Source: CAD feature listing. Evaluate the final solid. Frame: model axes, mm. Round coordinates to 2 decimals unless told otherwise and drop trailing zeros. Order: outer loops, then holes, each group sorted by start corner. A loop starts at its lowest first (then second) coordinate and runs counter-clockwise, first axis right, second up. Notation, with made-up numbers: M -12,5 L 39,5 A16 ccw 39,25 Z; hole C -12,47 d7. An arc over 180 degrees is marked long. Answer as CSV lines item,"result". Start each with the question number.
Item 1: Section query C-C on x = -110.5. Return the cut outline in (y, z), plus the area to 3 significant figures.
Item 2: Section query A-A on x = -41. Return the cut outline in (y, z), plus the area to 3 significant figures.
Item 3: Section query B-B on z = -5. Return the cut outline in (x, y), plus the area to 3 significant figures.
Item 4: First-contact query: P1, Ø3, axis at x = -23.5, z = 85, coming from the +Y side. Flat tip, straight axial feed; report the tip coordinate or a pass-through.
Item 5: Line query: line 1 (X direction, y = -2.25, z = 72); line 2 (X direction, y = -0.65, z = 65); line 3 (Z direction, x = -73, y = -1.25). Output: solid intervals per line, ascending. Write a range as [from, to].
from build123d import *

# Parameters (mm, degrees)
F1_DEPTH = 3
F2_DEPTH = 25
F3_R     = 20
F4_R     = 100
F5_R     = 15


with BuildPart() as f1:
    # F0 (on Front) → F1 (new body)
    with BuildSketch(Plane.XZ):
        with BuildLine():
            ThreePointArc((-119.2295857728, 16.5976797057), (-89.2269882152, -21.8866064143), (-44.5863344816, -2.1785326218))
            ThreePointArc((-44.5863344816, -2.1785326218), (-31.5003837254, 22.7075657451), (-18.8527258188, 47.819251244))
            ThreePointArc((-18.8527258187, 47.819251244), (-11.5073907558, 58.7139707042), (-8.9261215756, 71.5975225717))
            Line((-8.9261215756, 71.5975225717), (-11.67442069, 71.5975225717))
            Line((-11.67442069, 71.5975225717), (-11.67442069, 74.0203762137))
            ThreePointArc((-11.67442069, 74.0203762137), (-14.431706638, 81.8781100982), (-19.1607128584, 88.7325325952))
            ThreePointArc((-19.1607128584, 88.7325325952), (-48.5320541227, 98.3962580043), (-71.9061774941, 78.1548738354))
            Line((-71.9061774941, 78.1548738354), (-107.2845857728, 78.1548738354))
            Line((-107.2845857728, 78.1548738354), (-119.2295857728, 78.1548738354))
            Line((-119.2295857728, 78.1548738354), (-119.2295857728, 66.2098738354))
            Line((-119.2295857728, 66.2098738354), (-119.2295857728, 16.5976797057))
        make_face()
        with BuildLine():
            ThreePointArc((-26.6928125913, 79.0930187933), (-24.6315082315, 75.5227380173), (-23.3711215756, 71.597523888))
            Line((-23.3711215756, 71.597523888), (-20.8711215756, 71.5975236602))
            ThreePointArc((-20.8711215756, 71.5975236602), (-22.8939959961, 62.4935676044), (-28.5819229469, 55.1029300277))
            ThreePointArc((-28.5819229469, 55.1029300277), (-41.6104278008, 29.1671780434), (-55.1096433175, 3.4732809051))
            ThreePointArc((-55.1096433175, 3.4732809051), (-86.3130475025, -10.3024804429), (-107.2845857728, 16.5976797057))
            Line((-107.2845857728, 16.5976797057), (-107.2845857728, 66.2098738354))
            Line((-107.2845857728, 66.2098738354), (-104.7845857728, 66.2098738354))
            Line((-104.7845857728, 66.2098738354), (-68.5864427672, 66.2098738354))
            Line((-68.5864427672, 66.2098738354), (-63.1803487139, 66.2098738354))
            ThreePointArc((-63.1803487139, 66.2098738354), (-63.6941147242, 68.8812286524), (-63.8664115811, 71.5960777945))
            Line((-63.8664115811, 71.5960777945), (-61.3664115868, 71.5962461646))
            ThreePointArc((-61.3664115868, 71.5962461646), (-46.4685424734, 86.625019162), (-26.6928125913, 79.0930187933))
        make_face(mode=Mode.SUBTRACT)
        with BuildLine():
            ThreePointArc((-32.7025071715, 52.3956462756), (-51.243606048, 52.0172813271), (-63.1803487139, 66.2098738354))
            Line((-63.1803487139, 66.2098738354), (-68.5864427672, 66.2098738354))
            Line((-68.5864427672, 66.2098738354), (-104.7845857728, 66.2098738354))
            Line((-104.7845857728, 66.2098738354), (-104.7845857728, 16.5976797057))
            ThreePointArc((-104.7845857728, 16.5976797057), (-85.7031813006, -7.8780087034), (-57.3120938901, 4.6561636023))
            ThreePointArc((-57.3120938901, 4.6561636023), (-44.8056231456, 28.4219407394), (-32.7025071715, 52.3956462756))
        make_face()
        with BuildLine():
            ThreePointArc((-61.3664115868, 71.5962461646), (-42.368127741, 52.5998806027), (-23.3711215756, 71.597523888))
            Line((-23.3711215756, 71.597523888), (-28.5062876117, 71.7030383349))
            ThreePointArc((-28.5062876117, 71.7030383349), (-35.0280474509, 67.9936357913), (-42.4162418185, 66.6868830916))
            ThreePointArc((-42.4162418185, 66.6868830916), (-49.8149115034, 67.9342855665), (-56.3664115867, 71.5913571683))
            Line((-56.3664115866, 71.5913571683), (-61.3664115868, 71.5962461646))
        make_face()
        with BuildLine():
            ThreePointArc((-55.1096433175, 3.4732809051), (-41.6104278008, 29.1671780434), (-28.5819229469, 55.1029300277))
            ThreePointArc((-28.5819229469, 55.1029300277), (-30.5643455059, 53.6307678626), (-32.7025071715, 52.3956462756))
            ThreePointArc((-32.7025071715, 52.3956462756), (-44.8056231456, 28.4219407394), (-57.3120938901, 4.6561636023))
            ThreePointArc((-57.3120938901, 4.6561636023), (-85.7031813006, -7.8780087034), (-104.7845857728, 16.5976797057))
            Line((-104.7845857728, 16.5976797057), (-104.7845857728, 66.2098738354))
            Line((-104.7845857728, 66.2098738354), (-107.2845857728, 66.2098738354))
            Line((-107.2845857728, 66.2098738354), (-107.2845857728, 16.5976797057))
            ThreePointArc((-107.2845857728, 16.5976797057), (-86.3130475025, -10.3024804429), (-55.1096433175, 3.4732809051))
        make_face()
        with BuildLine():
            ThreePointArc((-42.4162418185, 66.6868830916), (-35.0280474509, 67.9936357913), (-28.5062876117, 71.7030383349))
            ThreePointArc((-28.5062876117, 71.7030383349), (-42.4756351565, 81.447422187), (-56.3664115866, 71.5913571682))
            ThreePointArc((-56.3664115867, 71.5913571683), (-49.8149115034, 67.9342855665), (-42.4162418185, 66.6868830916))
        make_face()
        with BuildLine():
            Line((-28.5062876117, 71.7030383349), (-23.3711215756, 71.597523888))
            ThreePointArc((-23.3711215756, 71.597523888), (-24.6315082315, 75.5227380173), (-26.6928125913, 79.0930187933))
            ThreePointArc((-26.6928125913, 79.0930187933), (-46.4685424734, 86.625019162), (-61.3664115868, 71.5962461646))
            Line((-61.3664115868, 71.5962461646), (-56.3664115866, 71.5913571683))
            ThreePointArc((-56.3664115866, 71.5913571682), (-42.4756351565, 81.447422187), (-28.5062876117, 71.7030383349))
        make_face()
        with BuildLine():
            Line((-20.8711215756, 71.5975236602), (-23.3711215756, 71.597523888))
            ThreePointArc((-23.3711215756, 71.597523888), (-42.368127741, 52.5998806027), (-61.3664115868, 71.5962461646))
            Line((-61.3664115868, 71.5962461646), (-63.8664115811, 71.5960777945))
            ThreePointArc((-63.8664115811, 71.5960777945), (-63.6941147242, 68.8812286524), (-63.1803487139, 66.2098738354))
            ThreePointArc((-63.1803487139, 66.2098738354), (-51.243606048, 52.0172813271), (-32.7025071715, 52.3956462756))
            ThreePointArc((-32.7025071715, 52.3956462756), (-30.5643455059, 53.6307678626), (-28.5819229469, 55.1029300277))
            ThreePointArc((-28.5819229469, 55.1029300277), (-22.8939959961, 62.4935676044), (-20.8711215756, 71.5975236602))
        make_face()
        with BuildLine():
            Line((-11.67442069, 71.5975225717), (-8.9261215756, 71.5975225717))
            ThreePointArc((-8.9261215756, 71.5975225717), (-13.1797411051, 80.6808937541), (-19.1607128584, 88.7325325952))
            ThreePointArc((-19.1607128584, 88.7325325952), (-14.431706638, 81.8781100982), (-11.67442069, 74.0203762137))
            Line((-11.67442069, 74.0203762137), (-11.67442069, 71.5975225717))
        make_face()
    extrude(amount=F1_DEPTH)

    # F0 (on Front) → F2 (cut)
    with BuildSketch(Plane.XZ):
        with BuildLine():
            ThreePointArc((-42.4162418185, 66.6868830916), (-35.0280474509, 67.9936357913), (-28.5062876117, 71.7030383349))
            ThreePointArc((-28.5062876117, 71.7030383349), (-42.4756351565, 81.447422187), (-56.3664115866, 71.5913571682))
            ThreePointArc((-56.3664115867, 71.5913571683), (-49.8149115034, 67.9342855665), (-42.4162418185, 66.6868830916))
        make_face()
    extrude(amount=F2_DEPTH, mode=Mode.SUBTRACT)

    # F3
    f3_edges = [f1.edges().sort_by_distance(p)[0] for p in [
        (-119.229586, -1.5, 78.154874),
    ]]
    fillet(f3_edges, radius=F3_R)

    # F4
    f4_edges = [f1.edges().sort_by_distance(p)[0] for p in [
        (-71.906177, -1.5, 78.154874),
    ]]
    fillet(f4_edges, radius=F4_R)

    # F5
    f5_edges = [f1.edges().sort_by_distance(p)[0] for p in [
        (-8.926122, -1.5, 71.597523),
    ]]
    fillet(f5_edges, radius=F5_R)


solid = f1.part
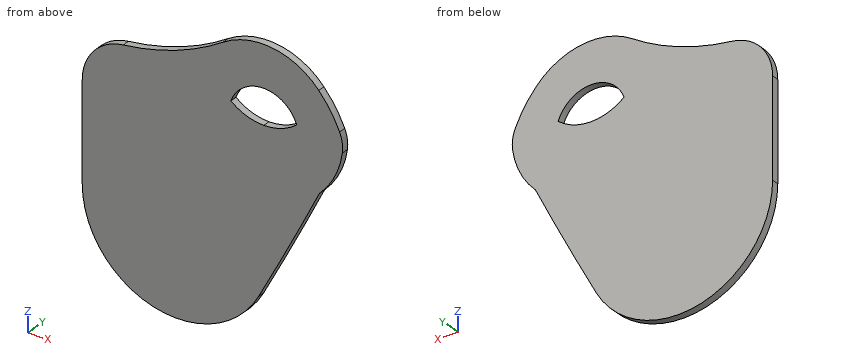
Results:
1,outline,"M -3,-8.23 L 0,-8.23 L 0,74.68 L -3,74.68 Z"
1,area,"249 mm^2"
2,outline,"M -3,4.54 L 0,4.54 L 0,66.74 L -3,66.74 Z; M -3,81.38 L 0,81.38 L 0,98.98 L -3,98.98 Z"
2,area,"239 mm^2"
3,outline,"M -112.84,-3 L -46.26,-3 L -46.26,0 L -112.84,0 Z"
3,area,"200 mm^2"
4,P1,"y = 0"
5,line 1,"[-113.66, -56.21], [-28.62, -9.35]"
5,line 2,"[-118.02, -9.58]"
5,line 3,"[-22.54, 86.35]"
